from build123d import *

# Parameters (mm, degrees)
SKETCH1_W                          = 12
SKETCH1_H                          = 10
SKETCH1_R                          = 1.5
BOSS_EXTRUDE1_DEPTH                = 24
SKETCH2_R                          = 1.754
SKETCH2_R_2                        = 1.5
BOSS_EXTRUDE2_DEPTH                = 0.5
TAP_DRILL_FOR_M1_6X0_35_TAP1_D     = 1.25
TAP_DRILL_FOR_M1_6X0_35_TAP1_DEPTH = 0.624460113
TAP_DRILL_FOR_M1_6X0_35_TAP1_TIP   = 0.375537887


with BuildPart() as part:
    # Sketch1 → Boss-Extrude1 (new body)
    with BuildSketch(Plane(origin=(0, 0, 0), x_dir=(1, 0, 0), z_dir=(0, 1, 0))):
        Rectangle(SKETCH1_W, SKETCH1_H)
        Circle(SKETCH1_R, mode=Mode.SUBTRACT)
    extrude(amount=BOSS_EXTRUDE1_DEPTH)

    # Sketch2 → Boss-Extrude2 (add)
    with BuildSketch(Plane.XZ):
        Circle(SKETCH2_R)
        Circle(SKETCH2_R_2, mode=Mode.SUBTRACT)
    extrude(amount=BOSS_EXTRUDE2_DEPTH)

    # Tap Drill for M1.6x0.35 Tap1
    with Locations(Plane(origin=(0, 0, 0), x_dir=(-1, 0, 0), z_dir=(0, -1, 0))):
        with Locations((-4.5, 0), (4.5, 0)):
            Hole(TAP_DRILL_FOR_M1_6X0_35_TAP1_D / 2, depth=TAP_DRILL_FOR_M1_6X0_35_TAP1_DEPTH)
            with Locations((0, 0, -(TAP_DRILL_FOR_M1_6X0_35_TAP1_DEPTH + TAP_DRILL_FOR_M1_6X0_35_TAP1_TIP / 2))):  # 118° drill point
                Cone(0, TAP_DRILL_FOR_M1_6X0_35_TAP1_D / 2, TAP_DRILL_FOR_M1_6X0_35_TAP1_TIP, mode=Mode.SUBTRACT)


solid = part.part
The model under review builds one solid part; all positions refer to its coordinate system, in mm. A direction names the side the tool comes from. Give positions to 0.01 mm unless a question says otherwise; leave off trailing zeros. Write each loop counter-clockwise with the first axis right and the second up, starting at its lowest first coordinate (ties: lowest second). Pieces come first, ordered by that corner, then holes.
1. For P1, Ø1, axis at x = 0.5, z = 3, coming from the -Y side, flat-tipped, find the tip position at first contact; note if it passes through.
2. Add section A-A, the plane x = 0. Write out the cut boundary in (y, z).
3. Draft analysis for pull direction X (two halves, no side actions). For faces 1 (the flat face through (0, 12, 5)), 2 (the flat face through (-6, 12, 0)), 3 (the cylindrical face through (-5.124, 0.317, -0.027)), 4 (the cylindrical face through (3.876, 0.317, -0.027)), state which applies: +X half, -X half, draft (parallel to the pull), parting line (faces both ways), or undercut.
4. Add section D-D, the plane x = -3.5. Write out the cut boundary in (y, z).
5. Add section C-C, the plane z = -4. Write out the cut boundary in (x, y).
6. Wall thickness on L1, parallel to X at y = 8, z = 0; L2, parallel to Y at x = -5.25, z = -1.5; L3, parallel to Z at x = 0, y = 8.25: over which ranges is each line inside the solid? List them lowest first.
7. Tool access review of faces 5 (the cylindrical face through (-1.5, 11.92, 0.07)), 6 (the cylindrical face through (-1.39, -0.25, -1.07)): name each direction out of +Z, -Z, +X, -X, +Y, -Y from which nothing blocks a thin tool from reaching the whole face with its end or side.
8. Add section B-B, the plane y = 5.5. Write out the cut boundary in (x, z), plus the area to 3 significant figures.
Worked answers:
1. P1: stops at y = 0
2. outline: (-0.5, -1.75) - (0, -1.75) - (0, -5) - (24, -5) - (24, -1.5) - (-0.5, -1.5) - close; (-0.5, 1.5) - (24, 1.5) - (24, 5) - (0, 5) - (0, 1.75) - (-0.5, 1.75) - close
3. face 1: draft
3. face 2: -X half
3. face 3: undercut
3. face 4: undercut
4. outline: (0, -5) - (24, -5) - (24, 5) - (0, 5) - close
5. outline: (-6, 0) - (6, 0) - (6, 24) - (-6, 24) - close
6. L1: x = -6 to -1.5, 1.5 to 6
6. L2: y = 0 to 24
6. L3: z = -5 to -1.5, 1.5 to 5
7. face 5: +Y, -Y
7. face 6: -Y
8. outline: (-6, -5) - (6, -5) - (6, 5) - (-6, 5) - close; hole circle Ø3 at (0, 0)
8. area: 113 mm2
